Read the model definition and answer for the solid it produces. Units are mm, in the model's axes. A direction names the side the tool comes from. Give positions to 0.01 mm unless a question says otherwise; leave off trailing zeros. Order: outer loops, then holes, each group sorted by start corner. A loop starts at its lowest first (then second) coordinate and runs counter-clockwise, first axis right, second up. Notation, with made-up numbers: (-19, 29) -> (9, 29) arc R14 ccw to (9, 37) -> close; hole circle Ø8 at (88.25, 89.5). An arc over 180 degrees is marked (long way). One line per item, written item: value. Start each with the question number.
from build123d import *

# Parameters (mm, degrees)
BOSS_EXTRUDE1_DEPTH         = 31.4
SKETCH2_W                   = 3
SKETCH2_H                   = 31.4
BOSS_EXTRUDE2_DEPTH         = 25
F_1_4_0_25_DIAMETER_HOLE1_D = 6.35


with BuildPart() as part:
    # Sketch1 → Boss-Extrude1 (new body)
    with BuildSketch(Plane(origin=(0, 0, 0), x_dir=(0, 0, -1), z_dir=(1, 0, 0))):
        Polygon((0, 0), (0, 20), (3, 20), (3, 3), (28.4, 3), (28.4, 20), (31.4, 20), (31.4, 0), align=None)
    extrude(amount=BOSS_EXTRUDE1_DEPTH)

    # Sketch2 → Boss-Extrude2 (add)
    with BuildSketch(Plane.XZ):
        with Locations((29.9, -15.7)):
            Rectangle(SKETCH2_W, SKETCH2_H)
        with Locations((1.5, -15.7)):
            Rectangle(SKETCH2_W, SKETCH2_H)
    extrude(amount=BOSS_EXTRUDE2_DEPTH)

    # 1/4 (0.25) Diameter Hole1 (through all)
    with Locations(Plane(origin=(31.4, 0, 0), x_dir=(0, 0, -1), z_dir=(1, 0, 0))):
        with Locations((15.7, -12.7)):
            Hole(F_1_4_0_25_DIAMETER_HOLE1_D / 2)


solid = part.part
Item 1: Find section B-B on z = -15.7. Write down the section's boundary in (x, y) (3 decimals).
Item 2: Find the intervals of material crossed by line 1 (Y direction, x = 2.3, z = -15.7) (3 decimals); line 2 (X direction, y = -16, z = -2); line 3 (Z direction, x = 24, y = 9.5), in increasing order. Write a range as from..to.
Item 3: Find section D-D on z = -8.5. Write down the section's boundary in (x, y).
Item 4: Flat-ended cylindrical pins translate along their axes: pin 1 (5.5 mm diameter, centred on y = -12.7, z = -15.7, fed in from -X) (3 decimals); pin 2 (7.5 mm diameter, centred on y = -12.7, z = -15.7, fed in from -X); pin 3 (1.5 mm diameter, centred on x = 11, z = -25.5, fed in from -Y); pin 4 (1 mm diameter, centred on x = 8.5, z = -19, fed in from +Y). Find the tip coordinate at first contact, or state that the pin passes through.
Item 5: Find section A-A on y = -12.7. Write down the section's boundary in (x, z) (3 decimals), then the cut area to 3 significant figures.
Item 6: For a pull along Z with two mould halves and no side action, classify faces 1 (the flat face through (15, 11, -28.4)), 2 (the cylindrical face through (29.88, -14.63, -18.22)), 3 (the flat face through (1, -25, -15)), 4 (the flat face through (15, 8, 0)) as +Z half, -Z half, draft (parallel to the pull), parting line (faces both ways), or undercut.
Item 7: Find section C-C on x = 17. Write down the section's boundary in (y, z).
Item 8: A tool of negligible diameter and unlimited length cuts with its end or side. For faces 5 (the flat face through (15, 8, -31.4)), 6 (the flat face through (15, 3, -16)), 7 (the flat face through (16, 0, -16)), from which of +Z, -Z, +X, -X, +Y, -Y can it reach the whole face along a straight path? Write none if from no direction.
Checks:
1. outline: (0, -25) -> (3, -25) -> (3, -15.875) -> (0, -15.875) -> close; (0, -9.525) -> (3, -9.525) -> (3, 0) -> (28.4, 0) -> (28.4, -9.525) -> (31.4, -9.525) -> (31.4, 3) -> (0, 3) -> close; (28.4, -25) -> (31.4, -25) -> (31.4, -15.875) -> (28.4, -15.875) -> close
2. line 1: -25..-15.875, -9.525..3
2. line 2: 0..3, 28.4..31.4
2. line 3: -31.4..-28.4, -3..0
3. outline: (0, -25) -> (3, -25) -> (3, 0) -> (28.4, 0) -> (28.4, -25) -> (31.4, -25) -> (31.4, 3) -> (0, 3) -> close
4. pin 1: through
4. pin 2: x = 0
4. pin 3: y = 0
4. pin 4: y = 3
5. outline: (0, -31.4) -> (3, -31.4) -> (3, -18.875) -> (0, -18.875) -> close; (0, -12.525) -> (3, -12.525) -> (3, 0) -> (0, 0) -> close; (28.4, -31.4) -> (31.4, -31.4) -> (31.4, -18.875) -> (28.4, -18.875) -> close; (28.4, -12.525) -> (31.4, -12.525) -> (31.4, 0) -> (28.4, 0) -> close
5. area: 150 mm2
6. face 1: undercut
6. face 2: undercut
6. face 3: draft
6. face 4: +Z half
7. outline: (0, -31.4) -> (20, -31.4) -> (20, -28.4) -> (3, -28.4) -> (3, -3) -> (20, -3) -> (20, 0) -> (0, 0) -> close
8. face 5: -Z, +X, -X, +Y, -Y
8. face 6: +X, -X, +Y
8. face 7: +Z, -Z, -Y
